Verification items for the finished model (mm, model axes). A direction names the side the tool comes from. Coordinates: 2 decimals unless noted, no trailing zeros. Loops run counter-clockwise (first coordinate to the right, second up) from the corner with the lowest first, then second, coordinate; pieces in that order, holes last.
Q1. Go/stop test with flat-tipped pins: P1, Ø3, axis at y = 3, z = 2.5, coming from the -X side; P2, Ø1, axis at x = -2.5, y = 2.5, coming from the -Z side. Record where each tip stops, or that it passes through.
Q2. Sectioned sample at C-C (y = 4.15). Enter the section's corners in (x, z) (3 decimals).
Q3. Material ranges on probe 1 along X at (y, z) = (2.55, 0); probe 2 along X at (y, z) = (2.15, 1.75); probe 3 along Z at (x, y) = (0.25, 3.2) (3 decimals), recorded low to high.
Q4. Access from +Z, -Z, +X, -X, +Y, -Y to the whole of each face (thin tool, end or side, straight path). Record for faces 1 (the face through (2.7, 3, 0.1)), 2 (the face through (0, 0, -2)).
Q5. Mould release check, pull along X, two halves, no side actions. Record for faces 3 (the face through (4.065, 2.958, -0.534)), 4 (the face through (0, 3, 1.875)), 5 (the face through (0, 6, -2)): +X half, -X half, draft (parallel to the pull), parting line (faces both ways), or undercut.
Q6. Sectioned sample at A-A (x = 0). Enter the section's corners in (y, z) (3 decimals).
Q7. Sectioned sample at D-D (z = 2.5). Enter the section's corners in (x, y), then the cut area to 3 significant figures.
Q8. Sectioned sample at B-B (z = 0). Enter the section's corners in (x, y).
```python
from build123d import *

# Parameters (mm, degrees)
SKETCH1_R           = 4.1
BOSS_EXTRUDE1_DEPTH = 6
CUT_EXTRUDE1_DEPTH  = 8


with BuildPart() as part:
    # Sketch1 → Boss-Extrude1 (new body)
    with BuildSketch(Plane(origin=(0, 0, 0), x_dir=(1, 0, 0), z_dir=(0, 1, 0))):
        with Locations(Location((0, 0, 0), (0, 0, 270))):
            Circle(SKETCH1_R)
    extrude(amount=BOSS_EXTRUDE1_DEPTH)

    # Sketch2 → Cut-Extrude1 (cut)
    with BuildSketch(Plane(origin=(0, 6, 0), x_dir=(1, 0, 0), z_dir=(0, 1, 0))):
        with BuildLine():
            Line((1.989817831, 1.825), (-1.989817831, 1.825))
            ThreePointArc((-1.989817831, 1.825), (-2.699781796, -0.034325722), (-1.942775077, -1.875))
            Line((-1.942775077, -1.875), (1.942775077, -1.875))
            ThreePointArc((1.942775077, -1.875), (2.699781796, -0.034325722), (1.989817831, 1.825))
        make_face()
    extrude(amount=-CUT_EXTRUDE1_DEPTH, mode=Mode.SUBTRACT)


solid = part.part
```
Geometry check:
1. P1: stops at x = -3.98
1. P2: stops at z = -3.58
2. outline: circle Ø8.2 at (0, 0); hole (-1.99, -1.825) - (1.99, -1.825) arc R2.7 ccw to (1.943, 1.875) - (-1.943, 1.875) arc R2.7 ccw to start
3. probe 1: x = -4.1 to -2.7, 2.7 to 4.1
3. probe 2: x = -3.71 to -2.06, 2.06 to 3.71
3. probe 3: z = -4.092 to -1.825, 1.875 to 4.092
4. face 1: +Y, -Y
4. face 2: +Z, -Z, +X, -X, -Y
5. face 3: parting line
5. face 4: undercut
5. face 5: draft
6. outline: (0, -4.1) - (6, -4.1) - (6, -1.825) - (0, -1.825) - close; (0, 1.875) - (6, 1.875) - (6, 4.1) - (0, 4.1) - close
7. outline: (-3.25, 0) - (3.25, 0) - (3.25, 6) - (-3.25, 6) - close
7. area: 39.0 mm2
8. outline: (-4.1, 0) - (-2.7, 0) - (-2.7, 6) - (-4.1, 6) - close; (2.7, 0) - (4.1, 0) - (4.1, 6) - (2.7, 6) - close
